Could you check a few things on this model? Use its own coordinates, in mm. A direction names the side the tool comes from. Round coordinates to 2 decimals unless told otherwise and drop trailing zeros. Order: outer loops, then holes, each group sorted by start corner. A loop starts at its lowest first (then second) coordinate and runs counter-clockwise, first axis right, second up. Notation, with made-up numbers: (47, 48) - (92, 48) arc R23 cw to (92, 81) - close; hole circle Ø9 at (-1, 2.5). An arc over 180 degrees is marked (long way). Use one line per item in the form item = value.
Solid Edge part; units mm, degrees
sketch "Sketch1" plane through (0, 0, 0) normal (0, -1, 0) x (1, 0, 0)
  line L0 (0, 0) -> (3.4, 0)
  arc A0 (3.4, 0) -> (4.25, -0.85) centre (3.4, -0.85) cw
  line L1 (4.25, -0.85) -> (4.25, -5)
  line L2 (4.25, -5) -> (2.5, -5)
  line L3 (2.5, -5) -> (2.5, -44.2)
  line L4 (2.5, -44.2) -> (1.7, -45)
  line L5 (1.7, -45) -> (0, -45)
revolve "RevolvedProtrusion1" add sketch "Sketch1" angle 360 about axis through (0, 0, -45) along (0, 0, 1)
sketch "Sketch2" plane through (0, 0, 0) normal (0, 0, 1) x (1, 0, 0)
  line L0 (-2, -1.1547) -> (-2, 1.1547)
  line L1 (-2, 1.1547) -> (0, 2.3094)
  line L2 (0, 2.3094) -> (2, 1.1547)
  line L3 (2, 1.1547) -> (2, -1.1547)
  line L4 (2, -1.1547) -> (0, -2.3094)
  line L5 (0, -2.3094) -> (-2, -1.1547)
extrude "Cutout1" cut sketch "Sketch2" against normal blind 2.5
sketch "Sketch3" plane through (0, 0, 0) normal (1, 0, 0) x (0, 1, 0)
  line L0 (0, -3.8333) -> (2.3094, -2.5)
  line L1 (0, -2.5) -> (2.3094, -2.5)
  line L2 (0, -2.5) -> (0, -3.8333)
revolve "RevolvedCutout1" cut sketch "Sketch3" angle 360 about axis through (0, 0, -60.325) along (0, 0, 1)
cosmetic_thread "Thread1"
properties part number "18"
Item 1: Will these pins go through, and if not, where does the flat tip stop? P1, Ø1.3, axis at x = 1, y = 2, coming from the -Z side; P2, Ø1.5, axis at x = 0.5, y = 0, coming from the +Z side; P3, Ø2, axis at x = 1, z = -18.5, coming from the -Y side; P4, Ø1.5, axis at y = -3, z = -35, coming from the +X side.
Found:
P1 = -45
P2 = -3.11
P3 = -2.5
P4 = 1.09
Item 2: I need wall thicknesses on L1, parallel to X at y = 1.5, z = -20.5; L2, parallel to Z at x = -3, y = -1.75. Which ranges of each line are inside material? Lowest first, please.
Found:
L1 = -2 to 2
L2 = -5 to 0
Item 3: For faces 1 (the face through (2, -2, -5)), 2 (the face through (2, 0, -1)), 3 (the face through (2.285, -3.584, -2.954)), which set-ups out of +Z, -Z, +X, -X, +Y, -Y let a thin tool reach every point of the face, with its end or its side?
Found:
face_1 = -Z
face_2 = +Z
face_3 = +Z, -Z
Item 4: If we mould it in two halves opening along X, with no side actions, what happens to faces 4 (the face through (1.014, -1.724, -1.232)), 5 (the face through (-1.014, 1.724, -1.232)), 6 (the face through (1, 2, 0)), 7 (the face through (-0.54, 2.44, -24.87))? For each: released by +X, released by -X, zero draft, split by the parting line, or undercut.
Found:
face_4 = undercut
face_5 = undercut
face_6 = zero draft
face_7 = split by the parting line
Item 5: Imagine slicing it at A-A on z = -34.5. Please give me the cut outline in (x, y), plus the area to 3 significant figures.
Found:
outline = circle Ø5 at (0, 0)
area = 19.6 mm2
